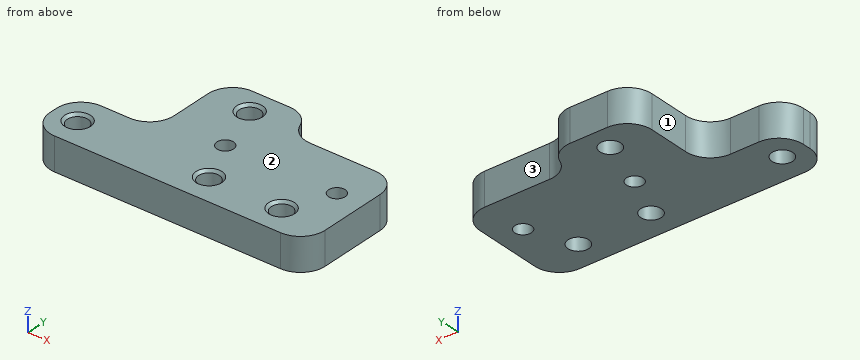
Autodesk Inventor part; units mm, degrees
ref_plane "YZ Plane" through (0, 0, 0) normal (1, 0, 0) x (0, 1, 0)
ref_plane "XZ Plane" through (0, 0, 0) normal (0, 1, 0) x (-1, 0, 0)
ref_plane "XY Plane" through (0, 0, 0) normal (0, 0, 1) x (1, 0, 0)
sketch "Sketch1" plane through (0, 0, 0) normal (0, 0, 1) x (1, 0, 0)
  line L0 (0, 0) -> (44, 0)
  line L1 (44, 0) -> (44, 22.5)
  line L2 (44, 22.5) -> (0, 22.5)
  line L3 (0, 22.5) -> (0, 0)
  line L4 (29, 5.5) -> (44, 5.5) construction
  line L5 (15, 5.5) -> (0, 5.5) construction
  line L6 (32.75, 14) -> (44, 14) construction
  line L7 (11.25, 14) -> (0, 14) construction
  line L8 (0, 11) -> (-15, 11)
  line L9 (-15, 11) -> (-15, 0)
  line L10 (-15, 0) -> (0, 0)
  line L11 (0, 0) -> (0, 11)
  line L12 (0, 22.5) -> (16, 22.5)
  line L13 (16, 22.5) -> (16, 28.5)
  line L14 (16, 28.5) -> (0, 28.5)
  line L15 (0, 28.5) -> (0, 22.5)
  line L16 (44, 5.5) -> (44, 22.5)
  point P0 (8, 23.8)
  point P1 (-10.3, 5.5)
  point P2 (-15, 5.5)
  point P3 (8, 28.5)
  dimension "d0" = 14
  dimension "d1" = 21.5
  dimension "d2" = 18.3
  dimension "d3" = 18.3
  dimension "d5" = 7
  dimension "d6" = 44
  dimension "d13" = 22.5
  dimension "d28" = 4.7
  dimension "d43" = 5.5
  dimension "d46" = 4.7
extrude "Extrusion1" add sketch "Sketch1" against normal blind 6.35
hole "Hole1" at (15, 5.5, 0) at (29, 5.5, 0) at (8, 23.8, 0) at (-10.3, 5.5, 0) direction (0, 0, -1) diameter 4 end through all countersink diameter 5 countersink angle 90
sketch "Sketch2" plane through (0, 0, 0) normal (0, 0, 1) x (1, 0, 0)
  line L0 (38, 26.3081) -> (49.0183, 26.3081)
  line L1 (49.0183, 26.3081) -> (49.0183, -7.071)
  line L2 (49.0183, -7.071) -> (38, -7.071)
  line L3 (38, -7.071) -> (38, 26.3081)
  line L4 (44, 0) -> (44, 22.5)
  point P0 (0, 0)
  dimension "d29" = 6
extrude "Extrusion2" cut sketch "Sketch2" against normal through all
hole "Hole2" at (11.25, 14, 0) at (32.75, 14, 0) direction (0, 0, -1) diameter 3.2 end through all
fillet "Fillet1" radius 4.75 8 edges at (38, 22.5, -3.175) (16, 28.5, -3.175) (0, 28.5, -3.175) (-15, 11, -3.175) (-15, 0, -3.175) (38, 0, -3.175) (0, 11, -3.175) (16, 22.5, -3.175)
properties part number "Hotend Mount"
Geometry: final body of the model. Coordinates: model frame, mm. Face numbers are marked on the shaded views. A direction names the side the tool comes from. Coordinates: 2 decimals unless noted, no trailing zeros. Loops run counter-clockwise (first coordinate to the right, second up) from the corner with the lowest first, then second, coordinate; pieces in that order, holes last. Notation, with made-up numbers: M -36,22.5 L -10,22.5 A34 cw -10,59.5 Z; hole C 48.25,-4 d8. An arc over 180 degrees is marked long. Put each result on its own line as item: value.
(1) First-contact query: pin 1 (3 mm diameter, centred on x = 18.5, z = -3.5, fed in from +Y); pin 2 (4.5 mm diameter, centred on x = 29, y = 5.5, fed in from +Z). Flat tips, straight axial feed; report the tip coordinate or a pass-through.
Answer sheet:
pin 1: stops at y = 24.33
pin 2: stops at z = -0.25
(2) Material intervals for probe 1 along X at (y, z) = (5.5, -3.1); probe 2 along Y at (x, z) = (32.75, -2.5); probe 3 along X at (y, z) = (14.75, -3.5), sorted ascending.
Answer sheet:
probe 1: x = -15 to -12.3, -8.3 to 13, 17 to 27, 31 to 38
probe 2: y = 0 to 12.4, 15.6 to 22.5
probe 3: x = -0.11 to 9.84, 12.66 to 31.34, 34.16 to 38
(3) Cut plane B-B on y = 5.5. Return the cut outline in (x, z), then the cut area to 3 significant figures.
Answer sheet:
outline: M -15,-6.35 L -12.3,-6.35 L -12.3,-0.5 L -12.8,0 L -15,0 Z; M -8.3,-6.35 L 13,-6.35 L 13,-0.5 L 12.5,0 L -7.8,0 L -8.3,-0.5 Z; M 17,-6.35 L 27,-6.35 L 27,-0.5 L 26.5,0 L 17.5,0 L 17,-0.5 Z; M 31,-6.35 L 38,-6.35 L 38,0 L 31.5,0 L 31,-0.5 Z
area: 260 mm^2
(4) Access query for the marked faces 1, 2 and 3. Directions: +Z, -Z, +X, -X, +Y, -Y. A direction counts if a zero-diameter tool reaches every point of the face in a straight line with its end or side. Return the directions, or none.
Answer sheet:
face 1: +Z, -Z, -X, +Y
face 2: +Z, +X, -X, +Y, -Y
face 3: +Z, -Z, +X, +Y
(5) Cut plane D-D on y = 14. Return the cut outline in (x, z).
Answer sheet:
outline: M -0.33,-6.35 L 9.65,-6.35 L 9.65,0 L -0.33,0 Z; M 12.85,-6.35 L 31.15,-6.35 L 31.15,0 L 12.85,0 Z; M 34.35,-6.35 L 38,-6.35 L 38,0 L 34.35,0 Z
(6) Cut plane A-A on x = 29. Return the cut outline in (y, z), then the cut area to 3 significant figures.
Answer sheet:
outline: M 0,-6.35 L 3.5,-6.35 L 3.5,-0.5 L 3,0 L 0,0 Z; M 7.5,-6.35 L 22.5,-6.35 L 22.5,0 L 8,0 L 7.5,-0.5 Z
area: 117 mm^2
(7) Cut plane C-C on x = 11.25. Return the cut outline in (y, z), then the cut area to 3 significant figures.
Answer sheet:
outline: M 0,-6.35 L 12.4,-6.35 L 12.4,0 L 0,0 Z; M 15.6,-6.35 L 28.5,-6.35 L 28.5,0 L 15.6,0 Z
area: 161 mm^2
